Solid Edge part; units mm, degrees
sketch "Sketch1" plane through (-29.1145, 0, 1.6522) normal (0, -1, 0) x (1, 0, 0)
  line L0 (30.4706, 13.7429) -> (36.4706, 13.7429)
  line L1 (30.4706, 15.7429) -> (30.4706, 13.7429)
  line L2 (32.9706, 15.7429) -> (30.4706, 15.7429)
  line L3 (32.9706, 14.7429) -> (32.9706, 15.7429)
  line L4 (33.7206, 14.7429) -> (32.9706, 14.7429)
  line L5 (33.7206, 15.7429) -> (33.7206, 14.7429)
  line L6 (34.7206, 15.7429) -> (33.7206, 15.7429)
  line L7 (34.7206, 14.7429) -> (34.7206, 15.7429)
  line L8 (35.4706, 14.7429) -> (34.7206, 14.7429)
  line L9 (35.4706, 15.7429) -> (35.4706, 14.7429)
  line L10 (36.4706, 15.7429) -> (35.4706, 15.7429)
  line L11 (36.4706, 13.7429) -> (36.4706, 15.7429)
extrude "Protrusion1" add sketch "Sketch1" against normal blind 13
properties material "Stainless Steel, 420"
Read the model definition and answer for the solid it produces. Units are mm, in the model's axes. A direction names the side the tool comes from. Give positions to 0.01 mm unless a question says otherwise; leave off trailing zeros. Order: outer loops, then holes, each group sorted by start corner. A loop starts at its lowest first (then second) coordinate and runs counter-clockwise, first axis right, second up.
(1) For faces 4 (the flat face through (4.606, 6, 17)), 5 (the flat face through (4, 0, 16)), determine the directions among +Z, -Z, +X, -X, +Y, -Y from which every point of the face is accessible in a straight line to the end or side of a thin tool.
(2) For a pull along X with two mould halves and no side action, classify faces 1 (the flat face through (5, 6, 17.395)), 2 (the flat face through (6.356, 6, 17)), 3 (the flat face through (1.356, 6, 16)) as released by +X, released by -X, zero draft, split by the parting line, or undercut.
(3) Find section C-C (x = 4.4). Give the vertices of the cut face in (y, z).
(4) Straight lines are drawn through the part: L1, parallel to X at y = 5, z = 16.9; L2, parallel to Z at x = 4.25, y = 9.5. For each, find the intervals that lie inside material, in ascending order.
(5) Find section B-B (y = 1.5). Give the vertices of the cut face in (x, z), plus the area to 3 significant figures.
(6) Find section A-A (z = 16.8). Give the vertices of the cut face in (x, y), plus the area to 3 significant figures.
Result sheet:
1. face 4: +Z, +Y, -Y
1. face 5: +Z, -Z, +X, -X, -Y
2. face 1: zero draft
2. face 2: undercut
2. face 3: released by -X
3. outline: (0, 15.4) - (13, 15.4) - (13, 16.4) - (0, 16.4) - close
4. L1: x = 1.36 to 3.86, 4.61 to 5.61, 6.36 to 7.36
4. L2: z = 15.4 to 16.4
5. outline: (1.36, 15.4) - (7.36, 15.4) - (7.36, 17.4) - (6.36, 17.4) - (6.36, 16.4) - (5.61, 16.4) - (5.61, 17.4) - (4.61, 17.4) - (4.61, 16.4) - (3.86, 16.4) - (3.86, 17.4) - (1.36, 17.4) - close
5. area: 10.5 mm2
6. outline: (1.36, 0) - (3.86, 0) - (3.86, 13) - (1.36, 13) - close; (4.61, 0) - (5.61, 0) - (5.61, 13) - (4.61, 13) - close; (6.36, 0) - (7.36, 0) - (7.36, 13) - (6.36, 13) - close
6. area: 58.5 mm2
